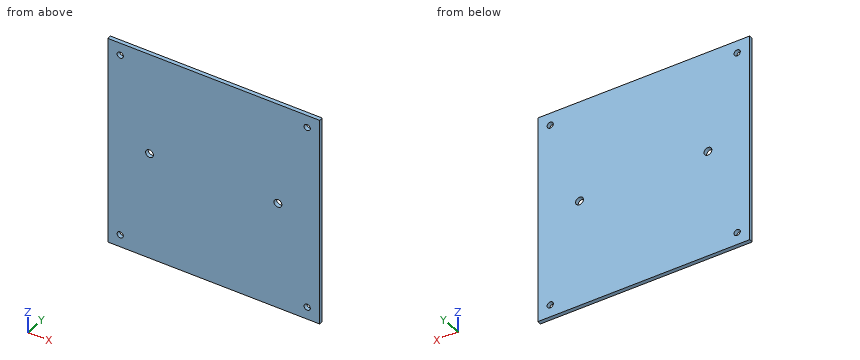
```python
from build123d import *

# Parameters (mm, degrees)
SKETCH1_W           = 170
SKETCH1_H           = 170
SKETCH1_R           = 2.5
SKETCH1_W_2         = 117
SKETCH1_H_2         = 122.5
SKETCH1_R_2         = 3.15
BOSS_EXTRUDE1_DEPTH = 3.175


with BuildPart() as part:
    # Sketch1 → Boss-Extrude1 (new body)
    # profile 1 of 2: a face of its own
    with BuildSketch(Plane(origin=(0, 0, 0), x_dir=(1, 0, 0), z_dir=(0, 1, 0))):
        Rectangle(SKETCH1_W, SKETCH1_H)
        with Locations(Location((75, -75, 0), (0, 0, 270))):
            Circle(SKETCH1_R, mode=Mode.SUBTRACT)
        with Locations(Location((75, 75, 0), (0, 0, 270))):
            Circle(SKETCH1_R, mode=Mode.SUBTRACT)
        with Locations(Location((-75, 75, 0), (0, 0, 270))):
            Circle(SKETCH1_R, mode=Mode.SUBTRACT)
        with Locations(Location((-75, -75, 0), (0, 0, 270))):
            Circle(SKETCH1_R, mode=Mode.SUBTRACT)
        Rectangle(SKETCH1_W_2, SKETCH1_H_2, mode=Mode.SUBTRACT)
    # profile 2 of 2: a face of its own
    with BuildSketch(Plane(origin=(0, 0, 0), x_dir=(1, 0, 0), z_dir=(0, 1, 0))):
        Rectangle(SKETCH1_W_2, SKETCH1_H_2)
        with Locations(Location((51.5, -2.25, 0), (0, 0, 270))):
            Circle(SKETCH1_R_2, mode=Mode.SUBTRACT)
        with Locations(Location((-51.5, -2.25, 0), (0, 0, 270))):
            Circle(SKETCH1_R_2, mode=Mode.SUBTRACT)
    extrude(amount=BOSS_EXTRUDE1_DEPTH)


solid = part.part
```
Part model, mm, in its own coordinate system. Round coordinates to 2 decimals unless told otherwise and drop trailing zeros. Loops run counter-clockwise (first coordinate to the right, second up) from the corner with the lowest first, then second, coordinate; pieces in that order, holes last. Notation, with made-up numbers: (89, 54) -> (121, 54) arc R16 cw to (121, 83) -> close; hole circle Ø3 at (60, 33). An arc over 180 degrees is marked (long way). Use CSV: the item, a comma, the result in double quotes. Start each with the question number.
1) Cut at B-B, the plane z = 75. Write the cut outline in (x, y) (3 decimals), plus the area to 3 significant figures.
2) Cut at C-C, the plane x = 51.5. Write the cut outline in (y, z) (3 decimals).
3) Wall check: L1, parallel to X at y = 1.2, z = 2.25; L2, parallel to X at y = 1.3, z = -75; L3, parallel to Z at x = 52.5, y = 0.7. Give the ranges that are in metal, low to high. Write a range as [from, to].
4) Cut at A-A, the plane x = -75. Write the cut outline in (y, z) (3 decimals).
Determined:
1,outline,"(-85, 0) -> (-77.5, 0) -> (-77.5, 3.175) -> (-85, 3.175) -> close; (-72.5, 0) -> (72.5, 0) -> (72.5, 3.175) -> (-72.5, 3.175) -> close; (77.5, 0) -> (85, 0) -> (85, 3.175) -> (77.5, 3.175) -> close"
1,area,"508 mm2"
2,outline,"(0, -85) -> (3.175, -85) -> (3.175, -0.9) -> (0, -0.9) -> close; (0, 5.4) -> (3.175, 5.4) -> (3.175, 85) -> (0, 85) -> close"
3,L1,"x = [-85, -54.65], [-48.35, 48.35], [54.65, 85]"
3,L2,"x = [-85, -77.5], [-72.5, 72.5], [77.5, 85]"
3,L3,"z = [-85, -0.74], [5.24, 85]"
4,outline,"(0, -85) -> (3.175, -85) -> (3.175, -77.5) -> (0, -77.5) -> close; (0, -72.5) -> (3.175, -72.5) -> (3.175, 72.5) -> (0, 72.5) -> close; (0, 77.5) -> (3.175, 77.5) -> (3.175, 85) -> (0, 85) -> close"
